Design review of the part built by this model. Coordinates are the model's own, in mm. A direction names the side the tool comes from. Give positions to 0.01 mm unless a question says otherwise; leave off trailing zeros. Loops run counter-clockwise (first coordinate to the right, second up) from the corner with the lowest first, then second, coordinate; pieces in that order, holes last. Notation, with made-up numbers: M -6.5,50.25 L 46.5,50.25 A24 ccw 46.5,80.25 Z; hole C -12,35.5 d5. An arc over 180 degrees is marked long. Use a Markdown table: item, result. Add a question column.
(1) Add section C-C, the plane x = -60. Give the boundary of the cut face in (y, z), then the cut area to 3 significant figures.
(2) For probe 1 along Y at (x, z) = (-75, 5); probe 2 along Y at (x, z) = (-60, 1.8); probe 3 along X at (y, z) = (-23.75, 2), list the stretches that pass through material, from the lowest coordinate up.
(3) Add section B-B, the plane z = 9. Give the boundary of the cut face in (x, y).
(4) Draft analysis for pull direction X (two halves, no side actions). For faces 1 (the face through (-60, -16, 5)), 2 (the face through (-60, -18.5, 6)), 3 (the face through (-50, -18, 5)), state which applies: pulls with the +X half, pulls with the -X half, needs draft (parallel to the pull), parting line crosses it, or undercut.
(5) Add section A-A, the plane x = -75. Give the boundary of the cut face in (y, z), then the cut area to 3 significant figures.
(6) Add section D-D, the plane y = -20. Give the boundary of the cut face in (x, z), then the cut area to 3 significant figures.
(7) For faces 4 (the face through (-65.66, -28.2, 6.55)), 5 (the face through (-70, -33, 5)), 6 (the face through (-50, -33, 5)), list the 3-axis set-ups (+Z, -Z, +X, -X, +Y, -Y) from which the entire face can be reached by the end or side of a thin tool; tool diameter is ignored.
(8) Insertion check: pin 1 Ø3 at (x, z) = (-73, 5.5) entering from +Y; pin 2 Ø3.5 at (y, z) = (-33, 6.5) entering from -X; pin 3 Ø2.5 at (y, z) = (-32.5, 3.5) entering from +X. Each pin has a flat end and moves straight along its axis. Give the tip position at first contact, or say it passes through.
```python
from build123d import *

# Parameters (mm, degrees)
SKETCH1_W           = 40
SKETCH1_H           = 12
SKETCH1_R           = 2
SKETCH1_R_2         = 4
BOSS_EXTRUDE1_DEPTH = 3
SKETCH2_W           = 20
SKETCH2_H           = 18
BOSS_EXTRUDE2_DEPTH = 7
SKETCH2_4_W         = 20
SKETCH2_4_H         = 18
BOSS_EXTRUDE3_DEPTH = 3
SKETCH3_W           = 10
SKETCH3_H           = 12
SKETCH3_R           = 2
BOSS_EXTRUDE4_DEPTH = 7
BOSS_EXTRUDE5_DEPTH = 3


with BuildPart() as part:
    # Sketch1 → Boss-Extrude1 (new body)
    with BuildSketch(Plane.XY):
        with Locations((-60, -25)):
            Rectangle(SKETCH1_W, SKETCH1_H)
        with Locations((-45, -25)):
            Circle(SKETCH1_R, mode=Mode.SUBTRACT)
        with Locations((-75, -25)):
            Circle(SKETCH1_R, mode=Mode.SUBTRACT)
        with Locations((-60, -25)):
            Circle(SKETCH1_R_2, mode=Mode.SUBTRACT)
    extrude(amount=BOSS_EXTRUDE1_DEPTH)

    # Sketch2 → Boss-Extrude2 (add)
    with BuildSketch(Plane.XY.offset(3)):
        with Locations((-60, -25)):
            Rectangle(SKETCH2_W, SKETCH2_H)
        Polygon((-56.24722325, -18.5), (-63.75277675, -18.5), (-67.505553499, -25), (-63.75277675, -31.5), (-56.24722325, -31.5), (-52.494446501, -25), align=None, mode=Mode.SUBTRACT)
    extrude(amount=BOSS_EXTRUDE2_DEPTH)

    # Sketch2<4> → Boss-Extrude3 (add)
    with BuildSketch(Plane.XY.offset(3)):
        with Locations((-60, -25)):
            Rectangle(SKETCH2_4_W, SKETCH2_4_H)
        Polygon((-56.24722325, -18.5), (-63.75277675, -18.5), (-67.505553499, -25), (-63.75277675, -31.5), (-56.24722325, -31.5), (-52.494446501, -25), align=None, mode=Mode.SUBTRACT)
    extrude(amount=-BOSS_EXTRUDE3_DEPTH)

    # Sketch3 → Boss-Extrude4 (add)
    # profile 1 of 6: a face of its own
    with BuildSketch(Plane.XY.offset(3)):
        Polygon((-50, -19), (-55.958548116, -19), (-52.494446501, -25), (-55.958548116, -31), (-50, -31), align=None)
    # profile 2 of 6: a face of its own
    with BuildSketch(Plane.XY.offset(3)):
        Polygon((-64.041451884, -31), (-70, -31), (-70, -34), (-50, -34), (-50, -31), (-55.958548116, -31), (-56.24722325, -31.5), (-63.75277675, -31.5), align=None)
    # profile 3 of 6: a face of its own
    with BuildSketch(Plane.XY.offset(3)):
        Polygon((-64.041451884, -19), (-70, -19), (-70, -31), (-64.041451884, -31), (-67.505553499, -25), align=None)
    # profile 4 of 6: a face of its own
    with BuildSketch(Plane.XY.offset(3)):
        Polygon((-70, -16), (-70, -19), (-64.041451884, -19), (-63.75277675, -18.5), (-56.24722325, -18.5), (-55.958548116, -19), (-50, -19), (-50, -16), align=None)
    # profile 5 of 6: a face of its own
    with BuildSketch(Plane.XY.offset(3)):
        with Locations((-75, -25)):
            Rectangle(SKETCH3_W, SKETCH3_H)
        with Locations((-75, -25)):
            Circle(SKETCH3_R, mode=Mode.SUBTRACT)
    # profile 6 of 6: a face of its own
    with BuildSketch(Plane.XY.offset(3)):
        with Locations((-45, -25)):
            Rectangle(SKETCH3_W, SKETCH3_H)
        with Locations((-45, -25)):
            Circle(SKETCH3_R, mode=Mode.SUBTRACT)
    extrude(amount=BOSS_EXTRUDE4_DEPTH)

    # Sketch3<4> → Boss-Extrude5 (add)
    with BuildSketch(Plane.XY.offset(3)):
        Polygon((-63.75277675, -18.5), (-64.041451884, -19), (-55.958548116, -19), (-56.24722325, -18.5), align=None)
        Polygon((-55.958548116, -31), (-64.041451884, -31), (-63.75277675, -31.5), (-56.24722325, -31.5), align=None)
    extrude(amount=-BOSS_EXTRUDE5_DEPTH)


solid = part.part
```
Established:
| question | item | result |
|---|---|---|
| 1 | outline | M -34,0 L -29,0 L -29,3 L -31.5,3 L -31.5,10 L -34,10 Z; M -21,0 L -16,0 L -16,10 L -18.5,10 L -18.5,3 L -21,3 Z |
| 1 | area | 65.0 mm^2 |
| 2 | probe 1 | -31 to -27, -23 to -19 |
| 2 | probe 2 | -34 to -29, -21 to -16 |
| 2 | probe 3 | -80 to -76.56, -73.44 to -63.8, -56.2 to -46.56, -43.44 to -40 |
| 3 | outline | M -80,-31 L -70,-31 L -70,-34 L -50,-34 L -50,-31 L -40,-31 L -40,-19 L -50,-19 L -50,-16 L -70,-16 L -70,-19 L -80,-19 Z; hole C -75,-25 d4; hole M -67.51,-25 L -63.75,-31.5 L -56.25,-31.5 L -52.49,-25 L -56.25,-18.5 L -63.75,-18.5 Z; hole C -45,-25 d4 |
| 4 | face 1 | needs draft |
| 4 | face 2 | undercut |
| 4 | face 3 | pulls with the +X half |
| 5 | outline | M -31,0 L -27,0 L -27,10 L -31,10 Z; M -23,0 L -19,0 L -19,10 L -23,10 Z |
| 5 | area | 80.0 mm^2 |
| 6 | outline | M -80,0 L -40,0 L -40,10 L -55.38,10 L -55.38,3 L -64.62,3 L -64.62,10 L -80,10 Z |
| 6 | area | 335 mm^2 |
| 7 | face 4 | +Z |
| 7 | face 5 | +Z, -Z, -X, -Y |
| 7 | face 6 | +Z, -Z, +X, -Y |
| 8 | pin 1 | y = -19 |
| 8 | pin 2 | x = -70 |
| 8 | pin 3 | x = -50 |
